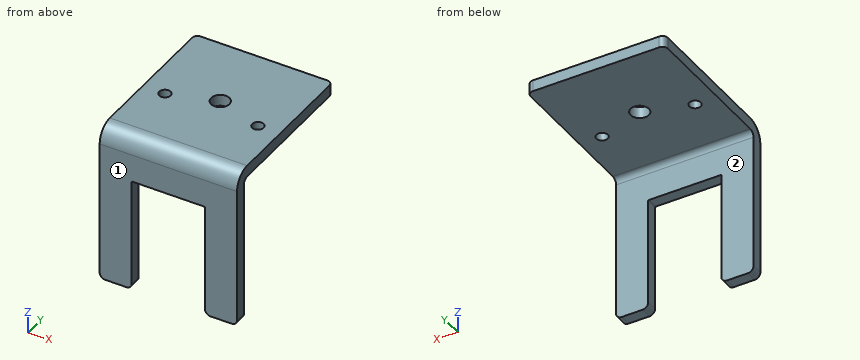
```python
from build123d import *

# Parameters (mm, degrees)
F1_DEPTH = 38.1
F3_DEPTH = 3.175
F4_R     = 1.524
F5_R     = 2.54
F5_R_2   = 1.5875
F6_DEPTH = 3.175
F7_W     = 70.9456168115
F7_H     = 45.830719173
F8_DEPTH = 19.05
F9_R     = 1.524


with BuildPart() as f1:
    # F0 (on Right) → F1 (new body)
    with BuildSketch(Plane.YZ):
        with BuildLine():
            Line((-64.0291666667, 0), (-60.8541666667, 0))
            Line((-60.8541666667, 0), (-60.8541666667, 39.243))
            ThreePointArc((-60.8541666667, 39.243), (-60.4077974012, 40.3206307345), (-59.3301666667, 40.767))
            Line((-59.3301666667, 40.767), (-0.5291666667, 40.767))
            Line((-0.5291666667, 40.767), (-0.5291666667, 43.942))
            Line((-0.5291666667, 43.942), (-59.3301666667, 43.942))
            ThreePointArc((-59.3301666667, 43.942), (-62.6528614315, 42.5656947648), (-64.0291666667, 39.243))
            Line((-64.0291666667, 39.243), (-64.0291666667, 0))
        make_face()
    extrude(amount=F1_DEPTH)

    # F2 (on face) → F3 (cut, through all)
    with BuildSketch(Plane.XZ.offset(64.0291666667)):
        with BuildLine():
            Line((8.89, 31.242), (8.89, 0))
            Line((8.89, 0), (29.21, 0))
            Line((29.21, 0), (29.21, 31.242))
            ThreePointArc((29.21, 31.242), (29.1356051224, 31.4216051224), (28.956, 31.496))
            Line((28.956, 31.496), (9.144, 31.496))
            ThreePointArc((9.144, 31.496), (8.9643948776, 31.4216051224), (8.89, 31.242))
        make_face()
    extrude(amount=-F3_DEPTH, mode=Mode.SUBTRACT)

    # F4
    f4_edges = [f1.edges().sort_by_distance(p)[0] for p in [
        (8.89, -62.441667, 0),
        (0, -62.441667, 0),
        (29.21, -62.441667, 0),
        (38.1, -62.441667, 0),
        (38.1, -0.529167, 42.3545),
        (0, -0.529167, 42.3545),
    ]]
    fillet(f4_edges, radius=F4_R)

    # F5 (on face) → F6 (cut, through all)
    with BuildSketch(Plane.XY.offset(43.942)):
        with Locations((19.05, -8.1491666667)):
            Circle(F5_R)
        with Locations((19.05, -39.8991666667)):
            Circle(F5_R)
        with Locations((31.9405, -44.0266666667)):
            Circle(F5_R_2)
        with Locations((6.1595, -44.0266666667)):
            Circle(F5_R_2)
    extrude(amount=-F6_DEPTH, mode=Mode.SUBTRACT)

    # F7 (on face) → F8 (cut)
    with BuildSketch(Plane(origin=(0, -0.5291666667, 0), x_dir=(-1, 0, 0), z_dir=(0, 1, 0))):
        with Locations((-19.1829390824, 42.4401424825)):
            Rectangle(F7_W, F7_H)
    extrude(amount=-F8_DEPTH, mode=Mode.SUBTRACT)

    # F9
    f9_edges = [f1.edges().sort_by_distance(p)[0] for p in [
        (38.1, -19.579167, 42.3545),
        (0, -19.579167, 42.3545),
    ]]
    fillet(f9_edges, radius=F9_R)


solid = f1.part
```
Build history of the part. All positions in model axes, mm. Face numbers are marked on the shaded views. A direction names the side the tool comes from. Coordinates: 2 decimals unless noted, no trailing zeros. Order: outer loops, then holes, each group sorted by start corner. A loop starts at its lowest first (then second) coordinate and runs counter-clockwise, first axis right, second up. Notation, with made-up numbers: (-30.5, 69) -> (6.5, 69) arc R33 cw to (6.5, 100) -> close; hole circle Ø3 at (56.5, 60). An arc over 180 degrees is marked (long way). Answer in a Markdown table with one row per item. Add a question column.
Q1. Drop flat-ended pins along their axis: pin 1 (12 mm diameter, centred on x = 17, y = -47.5, fed in from -Z); pin 2 (3 mm diameter, centred on x = 7, z = 37, fed in from +Y); pin 3 (2.5 mm diameter, centred on x = 17, y = -62, fed in from -Z). Give the stop position or say it passes through.
Q2. Band-saw the part on C-C, the plane y = -39. List the corners of the cut face in (x, z), then the cut area to 3 significant figures.
Q3. Band-saw the part on A-A, the plane z = 21. List the corners of the cut face in (x, y), then the cut area to 3 significant figures.
Q4. Wall check: line 1 along Z through (x, y) = (35.5, -53.5); line 2 along Y through (x, z) = (19.05, 42.2); line 3 along Y through (x, z) = (10.5, 38). Give the ranges that are in metal, low to high. Write a range as [from, to].
Q5. Band-saw the part on B-B, the plane x = 19.05. List the corners of the cut face in (y, z).
Q6. Which spindle directions (+Z, -Z, +X, -X, +Y, -Y) get a long thin tool onto all of the face, cutting with end or side? Do the marked faces 1 and 2. Say none if no direction does.
Q7. Band-saw the part on D-D, the plane z = 33.5. List the corners of the cut face in (x, y), then the cut area to 3 significant figures.
Answers follow:
| question | item | result |
|---|---|---|
| 1 | pin 1 | z = 40.77 |
| 1 | pin 2 | y = -60.85 |
| 1 | pin 3 | z = 31.5 |
| 2 | outline | (0, 40.77) -> (16.67, 40.77) -> (16.67, 43.94) -> (0, 43.94) -> close; (21.43, 40.77) -> (38.1, 40.77) -> (38.1, 43.94) -> (21.43, 43.94) -> close |
| 2 | area | 106 mm^2 |
| 3 | outline | (0, -64.03) -> (8.89, -64.03) -> (8.89, -60.85) -> (0, -60.85) -> close; (29.21, -64.03) -> (38.1, -64.03) -> (38.1, -60.85) -> (29.21, -60.85) -> close |
| 3 | area | 56.5 mm^2 |
| 4 | line 1 | [40.77, 43.94] |
| 4 | line 2 | [-62.98, -42.44], [-37.36, -19.58] |
| 4 | line 3 | [-64.03, -60.85] |
| 5 | outline | (-64.03, 31.5) -> (-60.85, 31.5) -> (-60.85, 39.24) arc R1.52 cw to (-59.33, 40.77) -> (-42.44, 40.77) -> (-42.44, 43.94) -> (-59.33, 43.94) arc R4.7 ccw to (-64.03, 39.24) -> close; (-37.36, 40.77) -> (-19.58, 40.77) -> (-19.58, 43.94) -> (-37.36, 43.94) -> close |
| 6 | face 1 | +Z, -Z, +X, -X, -Y |
| 6 | face 2 | -Z, +X, -X, +Y |
| 7 | outline | (0, -64.03) -> (38.1, -64.03) -> (38.1, -60.85) -> (0, -60.85) -> close |
| 7 | area | 121 mm^2 |
